Answer from the drawing. Dimensions are ordinates in mm from the lowest x, y and z of the part. Coordinates: 2 decimals unless noted, no trailing zeros. Order: outer loops, then holes, each group sorted by start corner. A loop starts at its lowest first (then second) coordinate and runs counter-clockwise, first axis right, second up.
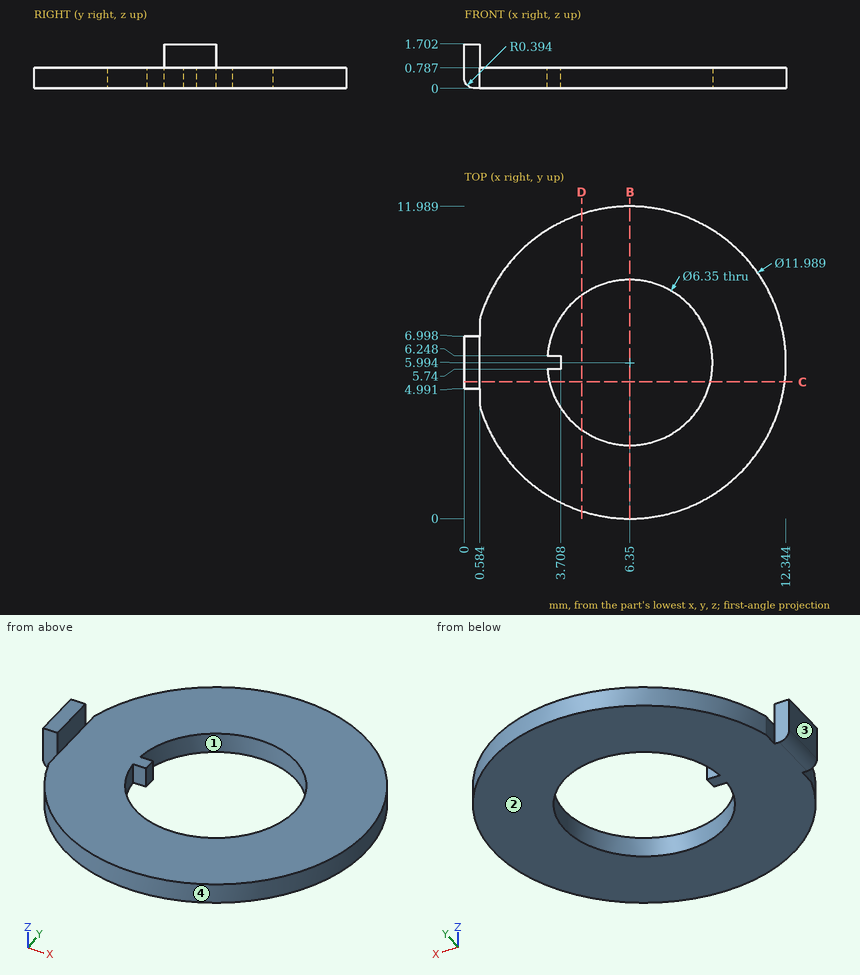
1) Section B-B (x = 6.35) is taken. Give the vertices of the cut face in (y, z).
2) Section C-C (y = 5.25) is taken. Give the vertices of the cut face in (x, z) (1 decimal).
3) Section D-D (x = 4.5) is taken. Give the vertices of the cut face in (y, z) (1 decimal).
4) Each of these flat-tipped pins is pushed along its axis until it touches: P1, Ø0.6, axis at x = 0, z = 1, coming from the -Y side; P2, Ø1, axis at x = 1.5, z = 0.5, coming from the -Y side; P3, Ø0.5, axis at x = 0.5, z = 1.5, coming from the +Y side. Where does it stop, or does it pass through?
5) Consider L1, parallel to Y at x = 6.35, z = 0.55; L2, parallel to Z at x = 9, y = 1.5; L3, parallel to X at y = 6, z = 1.15 (1 decimal). Determine where each line is inside the solid, lowest interval first.
6) Determine the mould class of the marked faces 1, 2, 3 and 4 for opening direction X: released by +X, released by -X, zero draft, split by the parting line, or undercut.
Filled sheet:
1. outline: (0, 0) - (2.82, 0) - (2.82, 0.79) - (0, 0.79) - close; (9.17, 0) - (11.99, 0) - (11.99, 0.79) - (9.17, 0.79) - close
2. outline: (0, 0.4) arc R0.4 ccw to (0.4, 0) - (3.3, 0) - (3.3, 0.8) - (0.6, 0.8) - (0.6, 1.7) - (0, 1.7) - close; (9.4, 0) - (12.3, 0) - (12.3, 0.8) - (9.4, 0.8) - close
3. outline: (0.3, 0) - (3.4, 0) - (3.4, 0.8) - (0.3, 0.8) - close; (8.6, 0) - (11.7, 0) - (11.7, 0.8) - (8.6, 0.8) - close
4. P1: stops at y = 4.99
4. P2: stops at y = 1.87
4. P3: stops at y = 7
5. L1: y = 0 to 2.82, 9.17 to 11.99
5. L2: z = 0 to 0.79
5. L3: x = 0 to 0.6
6. face 1: undercut
6. face 2: zero draft
6. face 3: released by -X
6. face 4: split by the parting line
